Autodesk Inventor part; units mm, degrees
ref_plane "YZ Plane" through (0, 0, 0) normal (1, 0, 0) x (0, 1, 0)
ref_plane "XZ Plane" through (0, 0, 0) normal (0, 1, 0) x (-1, 0, 0)
ref_plane "XY Plane" through (0, 0, 0) normal (0, 0, 1) x (1, 0, 0)
sketch "Эскиз1" plane through (0, 0, 0) normal (0, 0, 1) x (1, 0, 0)
  line L0 (-3, 300) -> (-3, 0)
  line L1 (-3, 0) -> (3, 0)
  line L2 (-3, 306) -> (-7.5, 306)
  line L3 (-7.5, 300) -> (-7.5, 306)
  line L4 (-7.5, 300) -> (-3, 300)
  line L5 (0, 0) -> (0, 306)
  line L6 (0, 306) -> (-3, 306)
  point P0 (0, 300)
  dimension "d1" = 3
  dimension "d4" = 7.5
  dimension "d6" = 6
  dimension "d8" = 300
revolve "Вращение1" add sketch "Эскиз1" angle 360 about axis through (0, 0, 0) along (0, 1, 0)
chamfer "Фаска1" distance 1 angle 45 1 edges at (3, 0, 0)
chamfer "Фаска2" distance 1 angle 45 2 edges at (7.5, 306, 0) (7.5, 300, 0)
thread "Резьба1"
equation "\"d1\" = 0.5 * d0"
equation "\"d4\" = 0.5 * d3"
properties part number "Шуп масло"
Geometry: final body of the model. Coordinates: model frame, mm. A direction names the side the tool comes from. Coordinates: 2 decimals unless noted, no trailing zeros. Order: outer loops, then holes, each group sorted by start corner. A loop starts at its lowest first (then second) coordinate and runs counter-clockwise, first axis right, second up.
1) Set-up query: faces 1 (the cylindrical face through (3, 148, 0)), 2 (the flat face through (0, 306, 0)). Return all of +Z, -Z, +X, -X, +Y, -Y with unobstructed straight access to the full face (end or side cutting, diameter ignored); none if empty.
Result sheet:
face 1: -Y
face 2: +Z, -Z, +X, -X, +Y
2) Section A-A (y = 119). Return loops of the section in (x, z), then the cut area to 3 significant figures.
Result sheet:
outline: circle Ø6 at (0, 0)
area: 28.3 mm2
3) First-contact query: P1, Ø3, axis at x = 2, y = 209, coming from the +Z side; P2, Ø3, axis at x = 2.5, z = -4, coming from the -Y side; P3, Ø1.5, axis at y = 57, z = -0.5, coming from the -X side. Flat tips, straight axial feed; report the tip coordinate or a pass-through.
Result sheet:
P1: stops at z = 2.96
P2: stops at y = 300
P3: stops at x = -3
4) Ray query, probe 1 along Y at (x, z) = (2.75, -3.5); probe 2 along X at (y, z) = (17, -0.5); probe 3 along Z at (x, y) = (1, 67.5). Return the intervals inside material, ascending.
Result sheet:
probe 1: y = 300 to 306
probe 2: x = -2.96 to 2.96
probe 3: z = -2.83 to 2.83
